Part model, mm, in its own coordinate system. A direction names the side the tool comes from. Give positions to 0.01 mm unless a question says otherwise; leave off trailing zeros. Write each loop counter-clockwise with the first axis right and the second up, starting at its lowest first coordinate (ties: lowest second). Pieces come first, ordered by that corner, then holes. Notation, with made-up numbers: M 62.25,0 L 68.25,0 A10 cw 68.25,17 Z; hole C 59,-15.75 d5. An arc over 180 degrees is marked long. Use CSV: the item, a comma, the result in double quotes. Start each with the question number.
1. Band-saw the part on B-B, the plane y = 0. List the corners of the cut face in (x, z), then the cut area to 3 significant figures.
2. Drill centre lines: line 1 along X through (y, z) = (-23.1, 0); line 2 along Y through (x, z) = (-14.5, -25); line 3 along Z through (x, y) = (-1, -19). Where is each one in solid material? Low to high. Write a range as from..to.
3. Drop flat-ended pins along their axis: pin 1 Ø6 at (x, z) = (-22, 0) entering from +Y; pin 2 Ø6 at (x, y) = (-9.5, -20) entering from +Z; pin 3 Ø4.5 at (x, y) = (-15.5, 15.5) entering from +Z. Give the stop position or say it passes through.
4. Mould opens along Z. For faces 1 (the face through (-15.4, -24, 5)), 2 (the face through (23.6, -24.46, 18.02)), 3 (the face through (-9, -9, -22)) say: pulls with the +Z half, pulls with the -Z half, needs draft (parallel to the pull), parting line crosses it, or undercut.
5. Band-saw the part on C-C, the plane z = 16. List the corners of the cut face in (x, y), then the cut area to 3 significant figures.
6. Band-saw the part on D-D, the plane x = 8. List the corners of the cut face in (y, z), then the cut area to 3 significant figures.
7. Band-saw the part on A-A, the plane z = 4. List the corners of the cut face in (x, y), then the cut area to 3 significant figures.
8. 3-axis set-ups, long thin cutter, end or side, ignore diameter. For faces 4 (the face through (0, -22, -15)), 5 (the face through (15.4, -24, 5)), 6 (the face through (-11.99, 0.53, -24.46)): which of +Z, -Z, +X, -X, +Y, -Y reach the whole face in a straight line?
from build123d import *

# Parameters (mm, degrees)
BOSS_EXTRUDE1_DEPTH = 25.4
SKETCH2_R           = 1.7
SKETCH2_R_2         = 12
CUT_EXTRUDE1_DEPTH  = 58.533989954
SKETCH4_W           = 30.8
SKETCH4_H           = 34
CUT_EXTRUDE2_DEPTH  = 58.533989954
SKETCH5_R           = 1.89865
CUT_EXTRUDE3_DEPTH  = 58.533989954
BOSS_EXTRUDE2_DEPTH = 3.9


with BuildPart() as part:
    # Sketch1 → Boss-Extrude1 (new, symmetric)
    with BuildSketch(Plane(origin=(0, 0, 0), x_dir=(0, 0, -1), z_dir=(1, 0, 0))):
        Polygon((-22, -22), (-22, -27), (27, -27), (27, 22), (22, 22), (22, -22), align=None)
    extrude(amount=BOSS_EXTRUDE1_DEPTH, both=True)

    # Sketch2 → Cut-Extrude1 (cut, through all)
    with BuildSketch(Plane.XY.offset(-22)):
        with Locations((-15.5, 15.5)):
            Circle(SKETCH2_R)
        with Locations((15.5, 15.5)):
            Circle(SKETCH2_R)
        with Locations((15.5, -15.5)):
            Circle(SKETCH2_R)
        with Locations((-15.5, -15.5)):
            Circle(SKETCH2_R)
        Circle(SKETCH2_R_2)
    extrude(amount=-CUT_EXTRUDE1_DEPTH, mode=Mode.SUBTRACT)

    # Sketch4 → Cut-Extrude2 (cut, through all)
    with BuildSketch(Plane(origin=(0, -22, 0), x_dir=(1, 0, 0), z_dir=(0, 1, 0))):
        with Locations((0, -5)):
            Rectangle(SKETCH4_W, SKETCH4_H)
    extrude(amount=-CUT_EXTRUDE2_DEPTH, mode=Mode.SUBTRACT)

    # Sketch5 → Cut-Extrude3 (cut, through all)
    with BuildSketch(Plane(origin=(0, -22, 0), x_dir=(1, 0, 0), z_dir=(0, 1, 0))):
        with Locations(Location((-22, 0, 0), (0, 0, 270))):
            Circle(SKETCH5_R)
        with Locations(Location((22, 0, 0), (0, 0, 270))):
            Circle(SKETCH5_R)
        with Locations(Location((22, -17, 0), (0, 0, 270))):
            Circle(SKETCH5_R)
        with Locations(Location((-22, -17, 0), (0, 0, 270))):
            Circle(SKETCH5_R)
    extrude(amount=-CUT_EXTRUDE3_DEPTH, mode=Mode.SUBTRACT)

    # Sketch6 → Boss-Extrude2 (add)
    with BuildSketch(Plane(origin=(25.4, 0, 0), x_dir=(0, 0, -1), z_dir=(1, 0, 0))):
        Polygon((22, 22), (5, -22), (22, -22), align=None)
    boss_extrude2 = extrude(amount=-BOSS_EXTRUDE2_DEPTH)

    # Mirror1: Boss-Extrude2 across plane
    add(boss_extrude2.mirror(Plane(origin=(0, 0, 0), x_dir=(0, 0, 1), z_dir=(1, 0, 0))))


solid = part.part
Output:
1,outline,"M -25.4,-27 L -12,-27 L -12,-22 L -21.5,-22 L -21.5,-13.5 L -25.4,-13.5 Z; M 12,-27 L 25.4,-27 L 25.4,-13.5 L 21.5,-13.5 L 21.5,-22 L 12,-22 Z"
1,area,"200 mm²"
2,line 1,"x = -25.4..-23.9, -20.1..-15.4, 15.4..20.1, 23.9..25.4"
2,line 2,"y = -27..-16.87, -14.13..14.13, 16.87..22"
2,line 3,"z = -27..-22"
3,pin 1,"stops at y = -22"
3,pin 2,"stops at z = -12"
3,pin 3,"stops at z = -22"
4,face 1,"needs draft"
4,face 2,"undercut"
4,face 3,"pulls with the +Z half"
5,outline,"M -25.4,-27 L -23.61,-27 L -23.61,-22 L -25.4,-22 Z; M -20.39,-27 L -15.4,-27 L -15.4,-22 L -20.39,-22 Z; M 15.4,-27 L 20.39,-27 L 20.39,-22 L 15.4,-22 Z; M 23.61,-27 L 25.4,-27 L 25.4,-22 L 23.61,-22 Z"
5,area,"67.7 mm²"
6,outline,"M -27,-27 L -8.94,-27 L -8.94,-22 L -22,-22 L -22,-12 L -27,-12 Z; M 8.94,-27 L 22,-27 L 22,-22 L 8.94,-22 Z"
6,area,"206 mm²"
7,outline,"M -25.4,-27 L -15.4,-27 L -15.4,-22 L -25.4,-22 Z; M 15.4,-27 L 25.4,-27 L 25.4,-22 L 15.4,-22 Z"
7,area,"100 mm²"
8,face 4,"+Z, +Y"
8,face 5,"+Z, +Y, -Y"
8,face 6,"+Z, -Z"
